Part print with two shaded views. Sizes in mm from the minimum x, y, z corner. Round coordinates to 2 decimals unless told otherwise and drop trailing zeros. Order: outer loops, then holes, each group sorted by start corner. A loop starts at its lowest first (then second) coordinate and runs counter-clockwise, first axis right, second up. Notation, with made-up numbers: M 9.25,49 L 38.25,49 A22 cw 38.25,88 Z; hole C 54.25,-20.5 d9. An arc over 180 degrees is marked long. One line per question, with ' | ' between items.
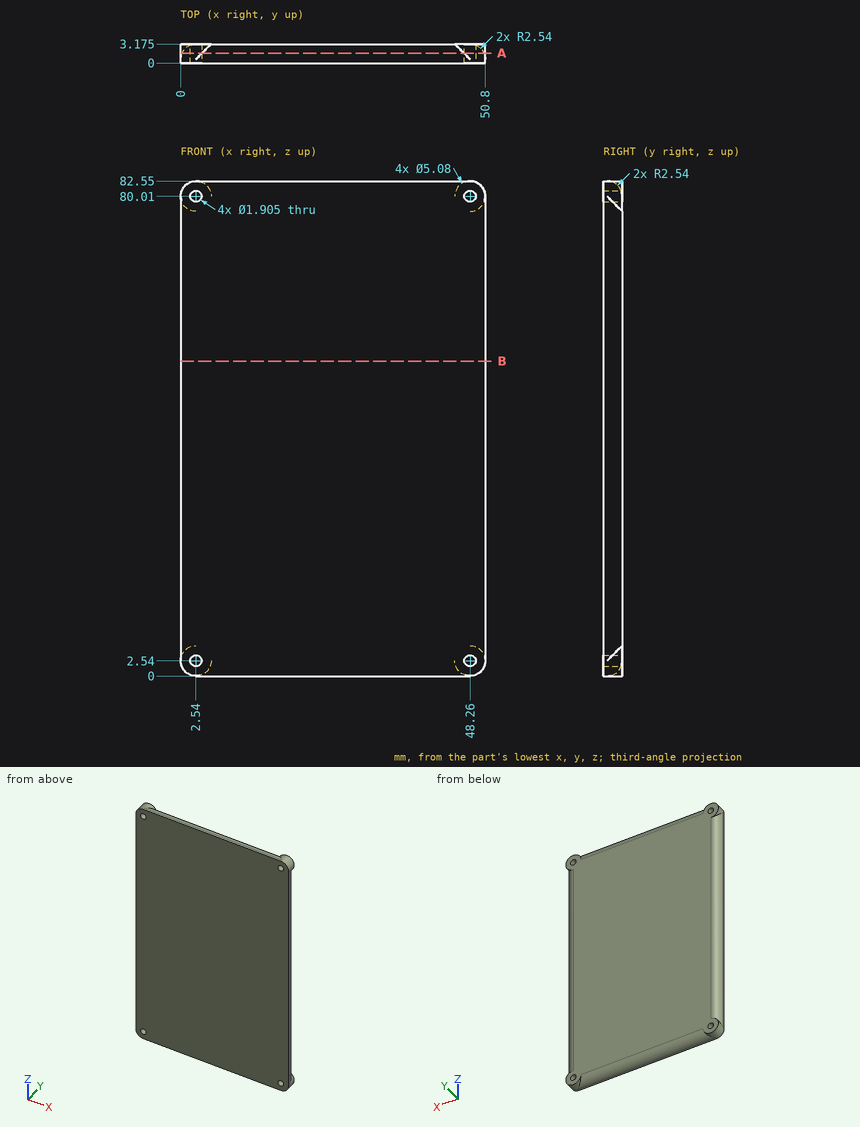
1) Saw through at B-B (z = 52.5). List the corners of the cut face in (x, y) (3 decimals).
The answers:
outline: M 0,0 L 50.8,0 L 50.8,0.635 A2.54 ccw 48.26,3.175 L 2.54,3.175 A2.54 ccw 0,0.635 Z
2) Saw through at A-A (y = 1.65). List the corners of the cut face in (x, z) (1 decimal).
The answers:
outline: M 0.2,3.6 A2.5 ccw 3.6,0.2 L 47.2,0.2 A2.5 ccw 50.6,3.6 L 50.6,79 A2.5 ccw 47.2,82.3 L 3.6,82.3 A2.5 ccw 0.2,79 Z; hole C 2.5,2.5 d1.9; hole C 2.5,80 d1.9; hole C 48.3,2.5 d1.9; hole C 48.3,80 d1.9
3) Drop flat-ended pins along their axis: pin 1 (1 mm diameter, centred on y = 2, z = 25, fed in from +X); pin 2 (1 mm diameter, centred on y = 1.5, z = 20.5, fed in from -X). Give the stop position or say it passes through.
The answers:
pin 1: stops at x = 50.65 | pin 2: stops at x = 0.03
4) Probe line 1 (Z direction, x = 2.54, y = 0.95); line 2 (X direction, y = 0.95, z = 80.01); line 3 (Z direction, x = 30.5, y = 0.95). List the from-to ranges inside material, lowest first. Write a range as [from, to].
The answers:
line 1: z = [0, 1.59], [3.49, 79.06], [80.96, 82.55] | line 2: x = [0, 1.59], [3.49, 47.31], [49.21, 50.8] | line 3: z = [0.02, 82.53]
